Can you work these out from the model? Positions are in its coordinate system, mm. Give positions to 0.01 mm unless a question says otherwise; leave off trailing zeros. Loops run counter-clockwise (first coordinate to the right, second up) from the corner with the lowest first, then second, coordinate; pieces in that order, holes last.
from build123d import *

# Parameters (mm, degrees)
F1_R     = 25
F2_DEPTH = 200


# Not quite as in the source:
# - a pattern or mirror of a feature is missing from the dataset's text; its kind, count and spacing are read off the source's solid


with BuildPart() as f2:
    # F1 (on Right) → F2 (new body, symmetric)
    with BuildSketch(Plane.YZ):
        Circle(F1_R)
    extrude(amount=F2_DEPTH, both=True)

    # F3 (on Front) → F4 (revolve)
    with BuildSketch(Plane.XZ):
        with BuildLine():
            add(Edge.make_bspline(
                [(200, 25), (199.201641866, 39.0983767897), (241.4136147213, 55.7899440033), (251.4561134334, 44.2516899933), (257.9215918294, 33.9973185388), (250, 13.5196693598), (250, 0)],
                knots=[0, 0, 0, 0, 0.3500294963, 0.535933113, 0.6975420206, 1, 1, 1, 1], degree=3))
            Line((200, 25), (200, 0))
            Line((200, 0), (250, 0))
        make_face()
    f4 = revolve(axis=Axis((225, 0, 0), (1, 0, 0)))

    # F4_copies: F4 across plane
    add(f4.mirror(Plane(origin=(0, 0, 0), x_dir=(0, 0, -1), z_dir=(-1, 0, 0))))


solid = f2.part
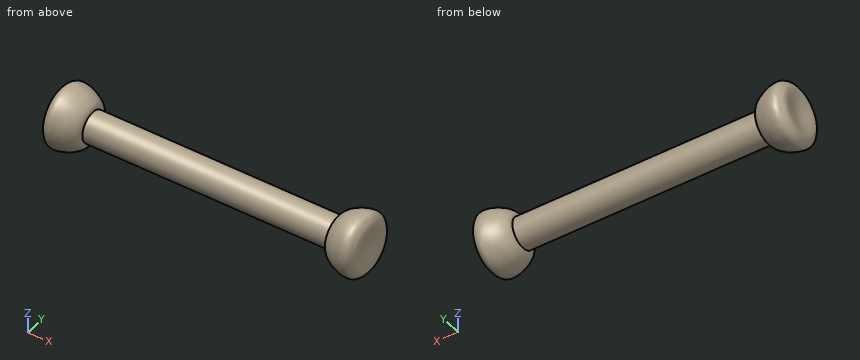
(1) Please list where these lines run through material, in increasing order: probe 1 along Z at (x, y) = (13, -2); probe 2 along X at (y, z) = (31.5, 2.5); probe 3 along X at (y, z) = (11.5, -25).
Returned:
probe 1: z = -24.92 to 24.92
probe 2: x = -254.85 to -201.68, 201.68 to 254.85
probe 3: x = -254.23 to -200.16, 200.16 to 254.23
(2) Suppose I cut it at A-A on x = -184. List the corners of the cut face in (y, z) for me, plus the area to 3 significant figures.
Returned:
outline: circle Ø50 at (0, 0)
area: 1,960 mm2
(3) Will these pins go through, and if not, where does the flat tip stop? P1, Ø3, axis at y = -32, z = -33.5, coming from the -X side; P2, Ø12, axis at y = -5.5, z = 2, coming from the +X side; P3, Ø3, axis at x = 97.5, y = 22, coming from the -Z side.
Returned:
P1: stops at x = -250.67
P2: stops at x = 251.09
P3: stops at z = -14.31
